from build123d import *

# Parameters (mm, degrees)
F0_W           = 105.41
F0_H           = 35.56
F0_R           = 1.5875
F1_DEPTH       = 5.969
F3_D           = 4.064
F3_DEPTH       = 50.8
F3_CSINK_D     = 7.874
F3_CSINK_ANGLE = 82


with BuildPart() as f1:
    # F0 (on Front) → F1 (new body)
    with BuildSketch(Plane.XZ):
        Rectangle(F0_W, F0_H)
        with Locations((-20.1295, 0)):
            Circle(F0_R, mode=Mode.SUBTRACT)
        with BuildLine():
            Line((-10.4775, 9.7155), (10.4775, 9.7155))
            ThreePointArc((10.4775, 9.7155), (12.722564, 8.785564), (13.6525, 6.5405))
            Line((13.6525, 6.5405), (13.6525, -6.5405))
            ThreePointArc((13.6525, -6.5405), (12.722564, -8.785564), (10.4775, -9.7155))
            Line((10.4775, -9.7155), (-10.4775, -9.7155))
            ThreePointArc((-10.4775, -9.7155), (-12.722564, -8.785564), (-13.6525, -6.5405))
            Line((-13.6525, -6.5405), (-13.6525, 6.5405))
            ThreePointArc((-13.6525, 6.5405), (-12.722564, 8.785564), (-10.4775, 9.7155))
        make_face(mode=Mode.SUBTRACT)
        with Locations((20.1295, 0)):
            Circle(F0_R, mode=Mode.SUBTRACT)
    extrude(amount=F1_DEPTH)

    # F3
    with Locations(Plane.XZ.offset(5.969)):
        with Locations((-48.5775, 13.716), (-48.5775, -13.716), (48.5775, -13.716), (48.5775, 13.716)):
            CounterSinkHole(F3_D / 2, F3_CSINK_D / 2, depth=F3_DEPTH, counter_sink_angle=F3_CSINK_ANGLE)


solid = f1.part
Read the model definition and answer for the solid it produces. Units are mm, in the model's axes. A direction names the side the tool comes from. Round coordinates to 2 decimals unless told otherwise and drop trailing zeros. Write each loop counter-clockwise with the first axis right and the second up, starting at its lowest first coordinate (ties: lowest second). Pieces come first, ordered by that corner, then holes. Notation, with made-up numbers: (55, 89) - (77, 89) arc R15 cw to (77, 100) - close; hole circle Ø2 at (-24.75, 76). An arc over 180 degrees is marked (long way). Use a Markdown table: item, result.
(1) The part is cut by section A-A (z = 0). Write down the section's boundary in (x, y) (1 decimal).
Reported:
| item | result |
|---|---|
| outline | (-52.7, -6) - (-21.7, -6) - (-21.7, 0) - (-52.7, 0) - close; (-18.5, -6) - (-13.7, -6) - (-13.7, 0) - (-18.5, 0) - close; (13.7, -6) - (18.5, -6) - (18.5, 0) - (13.7, 0) - close; (21.7, -6) - (52.7, -6) - (52.7, 0) - (21.7, 0) - close |
(2) Which of the six approach directions +Z, -Z, +X, -X, +Y, -Y give full straight-line access (tool end or side, diameter ignored) to faces 1 (the flat face through (0, -3, -9.716)), 2 (the conical face through (-48.1, -3.9, -15.8))?
Reported:
| item | result |
|---|---|
| face 1 | +Y, -Y |
| face 2 | -Y |
(3) The mould has two halves that part along Z. Classify faces 3 (the flat face through (-1, -3, -17.78)), 4 (the flat face through (-52.705, -3, 0)), 5 (the flat face through (-1, -3, 17.78)), 6 (the conical face through (48.9, -3.9, -11.6)): released by +Z, released by -Z, zero draft, split by the parting line, or undercut.
Reported:
| item | result |
|---|---|
| face 3 | released by -Z |
| face 4 | zero draft |
| face 5 | released by +Z |
| face 6 | undercut |
(4) The part is cut by section D-D (y = -2). State how many separate pieces and enclosed holes the cut face has, then the cut area to 3 significant figures.
Reported:
| item | result |
|---|---|
| separate pieces | 1 |
| enclosed holes | 7 |
| area | 3,160 mm2 |
(5) The part is cut by section C-C (x = -9). Write down the section's boundary in (y, z).
Reported:
| item | result |
|---|---|
| outline | (-5.97, -17.78) - (0, -17.78) - (0, -9.72) - (-5.97, -9.72) - close; (-5.97, 9.72) - (0, 9.72) - (0, 17.78) - (-5.97, 17.78) - close |
(6) The part is cut by section B-B (z = -4). Write down the section's boundary in (x, y) (1 decimal), then the cut area to 3 significant figures.
Reported:
| item | result |
|---|---|
| outline | (-52.7, -6) - (-13.7, -6) - (-13.7, 0) - (-52.7, 0) - close; (13.7, -6) - (52.7, -6) - (52.7, 0) - (13.7, 0) - close |
| area | 466 mm2 |
(7) This flat-tipped pin is pushed along its axis until it touches: pin 1 Ø4.5 at (x, z) = (-48.58, -13.72) entering from -Y. Where does it stop, or does it pass through?
Reported:
| item | result |
|---|---|
| pin 1 | y = -4.03 |
(8) Straight lines are drawn through the part: line 1 along X through (y, z) = (-3.2, 13.5) (3 decimals); line 2 along X through (y, z) = (-2.65, -6) (1 decimal); line 3 along Z through (x, y) = (1, -5.1). For each, find the intervals that lie inside material, in ascending order. Write a range as [from, to].
Reported:
| item | result |
|---|---|
| line 1 | [-52.705, -50.598], [-46.557, 46.557], [50.598, 52.705] |
| line 2 | [-52.7, -13.7], [13.7, 52.7] |
| line 3 | [-17.78, -9.72], [9.72, 17.78] |
